Source: CAD feature listing. Evaluate the final solid. Frame: model axes, mm. Face numbers are marked on the shaded views. A direction names the side the tool comes from. Coordinates: 2 decimals unless noted, no trailing zeros. Write each loop counter-clockwise with the first axis right and the second up, starting at its lowest first coordinate (ties: lowest second). Pieces come first, ordered by that corner, then holes. Notation, with made-up numbers: M 26,70 L 73,70 A21 cw 73,81 Z; hole C 4,-13 d7. An arc over 180 degrees is marked long. One line per item, written item: value. Start each with the question number.
Item 1: Mould query, pull axis X, two halves, no side actions, for the marked faces 3, 4, 5 and 6. Classes: released by +X, released by -X, zero draft, split by the parting line, or undercut.
Item 2: Set-up query: the marked faces 1 and 2. Return all of +Z, -Z, +X, -X, +Y, -Y with unobstructed straight access to the full face (end or side cutting, diameter ignored); none if empty.
Item 3: Cut plane B-B, the plane y = -37. Output: boundary loops of the cut face in (x, z), then the cut area to 3 significant figures.
Item 4: Pin query (flat end, axial travel): P1, Ø1, axis at x = 122, y = -49.5, coming from the -Z side; P2, Ø3.5, axis at x = 134, y = 49, coming from the +Z side; P3, Ø1.5, axis at x = 120, y = -50.5, coming from the -Z side; P4, Ø8, axis at x = 14.5, y = -31.5, coming from the -Z side. Return the tip coordinate at first contact, or that it passes through.
Item 5: Ray query, L1, parallel to X at y = 0, z = -105.3; L2, parallel to X at y = 0.5, z = -114; L3, parallel to Y at x = -134, z = -97.95. Return the intervals inside material, ascending. Write a range as from..to.
Item 6: Cut plane A-A, the plane x = -78.5. Output: boundary loops of the cut face in (y, z).
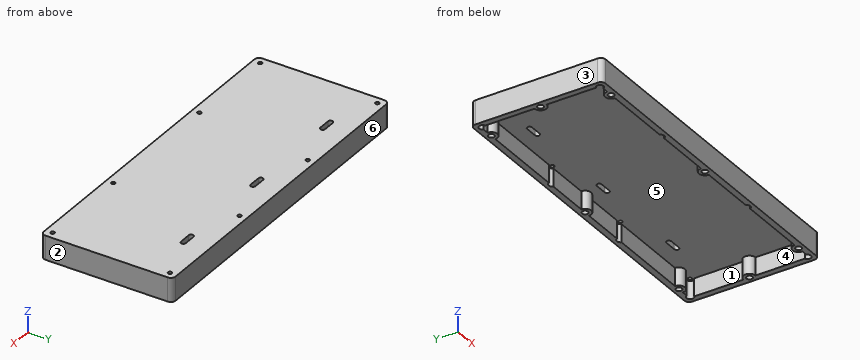
```python
from build123d import *

# Parameters (mm, degrees)
SKETCH022_R     = 1.6
PAD008_DEPTH    = 5
PAD009_DEPTH    = 15
SKETCH024_R     = 2.5
POCKET014_DEPTH = 6.5
SKETCH025_R     = 1.6
POCKET015_DEPTH = 5


with BuildPart() as part:
    # Sketch022 (on ShapeBinder) → Pad008 (new body)
    with BuildSketch(Plane(origin=(0, 0, -95), x_dir=(1, 0, 0), z_dir=(0, 0, -1))):
        with BuildLine():
            Line((-136, 55), (136, 55))
            ThreePointArc((140, 51), (138.828427, 53.828427), (136, 55))
            Line((140, -51), (140, 51))
            ThreePointArc((136, -55), (138.828427, -53.828427), (140, -51))
            Line((-136, -55), (136, -55))
            ThreePointArc((-140, -51), (-138.828427, -53.828427), (-136, -55))
            Line((-140, 51), (-140, -51))
            ThreePointArc((-136, 55), (-138.828427, 53.828427), (-140, 51))
        make_face()
        with Locations((134, 49)):
            Circle(SKETCH022_R, mode=Mode.SUBTRACT)
        with Locations((134, -49)):
            Circle(SKETCH022_R, mode=Mode.SUBTRACT)
        with Locations((44, -49)):
            Circle(SKETCH022_R, mode=Mode.SUBTRACT)
        with Locations((-44, -49)):
            Circle(SKETCH022_R, mode=Mode.SUBTRACT)
        with Locations((-134, -49)):
            Circle(SKETCH022_R, mode=Mode.SUBTRACT)
        with Locations((-134, 49)):
            Circle(SKETCH022_R, mode=Mode.SUBTRACT)
        with Locations((-55.592233, 49)):
            Circle(SKETCH022_R, mode=Mode.SUBTRACT)
        with Locations((55.592233, 49)):
            Circle(SKETCH022_R, mode=Mode.SUBTRACT)
        with BuildLine():
            ThreePointArc((-95, -33), (-97, -35), (-95, -37))
            Line((-95, -37), (-85, -37))
            ThreePointArc((-85, -37), (-83, -35), (-85, -33))
            Line((-95, -33), (-85, -33))
        make_face(mode=Mode.SUBTRACT)
        with BuildLine():
            ThreePointArc((-5, -33), (-7, -35), (-5, -37))
            Line((-5, -37), (5, -37))
            ThreePointArc((5, -37), (7, -35), (5, -33))
            Line((-5, -33), (5, -33))
        make_face(mode=Mode.SUBTRACT)
        with BuildLine():
            ThreePointArc((85, -33), (83, -35), (85, -37))
            Line((85, -37), (95, -37))
            ThreePointArc((95, -37), (97, -35), (95, -33))
            Line((85, -33), (95, -33))
        make_face(mode=Mode.SUBTRACT)
    extrude(amount=PAD008_DEPTH)

    # Sketch023 (on Face30 of Pad008) → Pad009 (join)
    with BuildSketch(Plane(origin=(0, 0, -100), x_dir=(1, 0, 0), z_dir=(0, 0, -1))):
        with BuildLine():
            Line((-136, 55), (136, 55))
            ThreePointArc((140, 51), (138.828427, 53.828427), (136, 55))
            Line((140, 51), (140, -51))
            ThreePointArc((136, -55), (138.828427, -53.828427), (140, -51))
            Line((136, -55), (-136, -55))
            ThreePointArc((-140, -51), (-138.828427, -53.828427), (-136, -55))
            Line((-140, -51), (-140, 51))
            ThreePointArc((-136, 55), (-138.828427, 53.828427), (-140, 51))
        make_face()
        with BuildLine():
            ThreePointArc((-46.828427, -50), (-44, -52), (-41.171573, -50))
            Line((-41.171573, -50), (-5, -50))
            ThreePointArc((5, -50), (0, -45), (-5, -50))
            Line((41.171573, -50), (5, -50))
            ThreePointArc((41.171573, -50), (44, -52), (46.828427, -50))
            Line((46.828427, -50), (116.171573, -50))
            ThreePointArc((126.171573, -50), (121.171573, -45), (116.171573, -50))
            Line((131.171573, -50), (126.171573, -50))
            ThreePointArc((131.171573, -50), (136.12132, -51.12132), (135, -46.171573))
            Line((135, -46.171573), (135, -5))
            ThreePointArc((135, 5), (130, 0), (135, -5))
            Line((135, 46.171573), (135, 5))
            ThreePointArc((135, 46.171573), (136.12132, 51.12132), (131.171573, 50))
            Line((131.171573, 50), (126.171573, 50))
            ThreePointArc((116.171573, 50), (121.171573, 45), (126.171573, 50))
            Line((58.42066, 50), (116.171573, 50))
            ThreePointArc((58.42066, 50), (55.592233, 52), (52.763806, 50))
            Line((52.763806, 50), (5, 50))
            ThreePointArc((-5, 50), (0, 45), (5, 50))
            Line((-52.763806, 50), (-5, 50))
            ThreePointArc((-52.763806, 50), (-55.592233, 52), (-58.42066, 50))
            Line((-58.42066, 50), (-116.171573, 50))
            ThreePointArc((-126.171573, 50), (-121.171573, 45), (-116.171573, 50))
            Line((-131.171573, 50), (-126.171573, 50))
            ThreePointArc((-131.171573, 50), (-136.12132, 51.12132), (-135, 46.171573))
            Line((-135, 46.171573), (-135, 5))
            ThreePointArc((-135, -5), (-130, 0), (-135, 5))
            Line((-135, -46.171573), (-135, -5))
            ThreePointArc((-135, -46.171573), (-136.12132, -51.12132), (-131.171573, -50))
            Line((-131.171573, -50), (-126.171573, -50))
            ThreePointArc((-116.171573, -50), (-121.171573, -45), (-126.171573, -50))
            Line((-46.828427, -50), (-116.171573, -50))
        make_face(mode=Mode.SUBTRACT)
    extrude(amount=PAD009_DEPTH)

    # Sketch024 (on Face33 of Pad009) → Pocket014 (cut)
    with BuildSketch(Plane(origin=(0, 0, -115), x_dir=(1, 0, 0), z_dir=(0, 0, -1))):
        with Locations((-121.171573, 50)):
            Circle(SKETCH024_R)
        with Locations((0, 50)):
            Circle(SKETCH024_R)
        with Locations((121.171573, 50)):
            Circle(SKETCH024_R)
        with Locations((-135, 0)):
            Circle(SKETCH024_R)
        with Locations((-121.171573, -50)):
            Circle(SKETCH024_R)
        with Locations((0, -50)):
            Circle(SKETCH024_R)
        with Locations((121.171573, -50)):
            Circle(SKETCH024_R)
        with Locations((135, 0)):
            Circle(SKETCH024_R)
    extrude(amount=-POCKET014_DEPTH, mode=Mode.SUBTRACT)

    # Sketch025 (on Face83 of Pocket014) → Pocket015 (cut)
    with BuildSketch(Plane(origin=(0, 0, -108.5), x_dir=(1, 0, 0), z_dir=(0, 0, -1))):
        with Locations((-121.171573, 50)):
            Circle(SKETCH025_R)
        with Locations((-135, 0)):
            Circle(SKETCH025_R)
        with Locations((0, 50)):
            Circle(SKETCH025_R)
        with Locations((-121.171573, -50)):
            Circle(SKETCH025_R)
        with Locations((0, -50)):
            Circle(SKETCH025_R)
        with Locations((121.171573, -50)):
            Circle(SKETCH025_R)
        with Locations((135, 0)):
            Circle(SKETCH025_R)
        with Locations((121.171573, 50)):
            Circle(SKETCH025_R)
    extrude(amount=-POCKET015_DEPTH, mode=Mode.SUBTRACT)


solid = part.part
```
From the geometry:
1. face 3: released by -X
1. face 4: undercut
1. face 5: undercut
1. face 6: zero draft
2. face 1: -Z
2. face 2: +Z, -Z, +X, +Y, -Y
3. outline: M -140,-115 L -135,-115 L -135,-100 L 135,-100 L 135,-115 L 140,-115 L 140,-95 L -140,-95 Z
3. area: 1,550 mm²
4. P1: stops at z = -103.5
4. P2: stops at z = -95
4. P3: stops at z = -108.5
4. P4: stops at z = -100
5. L1: x = -140..-136.6, -133.4..-130, 130..133.4, 136.6..140
5. L2: x = -140..-137.45, -132.55..-130.03, 130.03..132.55, 137.45..140
5. L3: y = -55..-50.6, -47.4..47.4, 50.6..55
6. outline: M -55,-115 L -50,-115 L -50,-100 L 50,-100 L 50,-115 L 55,-115 L 55,-95 L -55,-95 Z
